Design review of the part shown in the three views and the two pictorial views. Dimensions are in mm from the part's minimum x, y and z. A direction names the side the tool comes from. Give positions to 0.01 mm unless a question says otherwise; leave off trailing zeros. Loops run counter-clockwise (first coordinate to the right, second up) from the corner with the lowest first, then second, coordinate; pieces in that order, holes last. Notation, with made-up numbers: (42.5, 64.5) -> (99.5, 64.5) arc R10 ccw to (99.5, 81.5) -> close; hole circle Ø9 at (4, -34). An arc over 180 degrees is marked (long way). Answer as CSV lines item,"result".
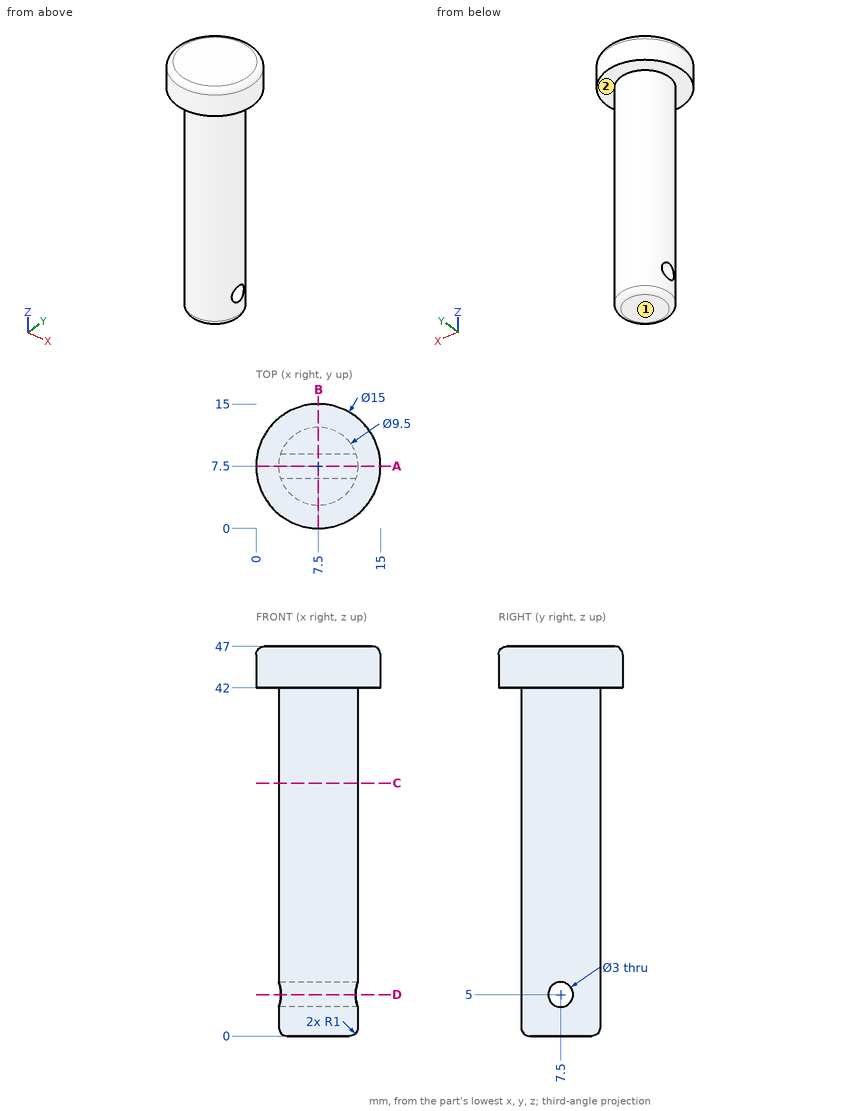
Q1. To check wall thickness, follow probe 1 along Z at (x, y) = (8, 7.5); probe 2 along Y at (x, z) = (7.75, 5); probe 3 along Y at (x, z) = (7.75, 23). State the ranges of each line that lie inside material, in increasing order. Write a range as from..to.
Filled sheet:
probe 1,"z = 0..3.5, 6.5..47"
probe 2,"y = 2.76..6, 9..12.24"
probe 3,"y = 2.76..12.24"
Q2. We need section C-C, the plane z = 30.5. State the section outline as (x, y) points, and give its area (3 significant figures).
Filled sheet:
outline,"circle Ø9.5 at (7.5, 7.5)"
area,"70.9 mm^2"
Q3. We need section A-A, the plane y = 7.5. State the section outline as (x, z) points, and give its area (3 significant figures).
Filled sheet:
outline,"(0, 42) -> (2.75, 42) -> (2.75, 6.5) -> (12.25, 6.5) -> (12.25, 42) -> (15, 42) -> (15, 46) arc R1 ccw to (14, 47) -> (1, 47) arc R1 ccw to (0, 46) -> close; (2.75, 1) arc R1 ccw to (3.75, 0) -> (11.25, 0) arc R1 ccw to (12.25, 1) -> (12.25, 3.5) -> (2.75, 3.5) -> close"
area,"445 mm^2"
Q4. We need section B-B, the plane x = 7.5. State the section outline as (y, z) points.
Filled sheet:
outline,"(0, 42) -> (2.75, 42) -> (2.75, 1) arc R1 ccw to (3.75, 0) -> (11.25, 0) arc R1 ccw to (12.25, 1) -> (12.25, 42) -> (15, 42) -> (15, 46) arc R1 ccw to (14, 47) -> (1, 47) arc R1 ccw to (0, 46) -> close; hole circle Ø3 at (7.5, 5)"
Q5. Clearance check with flat-ended pins moving along their axes: pin 1 Ø6 at (y, z) = (3.5, 8.5) entering from +X; pin 2 Ø5 at (x, z) = (12, 17) entering from -Y; pin 3 Ø6 at (y, z) = (8.5, 17) entering from +X; pin 4 Ø2.5 at (y, z) = (7.5, 5) entering from -X. State where each tip first meets the part, or that it passes through.
Filled sheet:
pin 1,"stops at x = 12.14"
pin 2,"stops at y = 3.19"
pin 3,"stops at x = 12.25"
pin 4,"passes through"
Q6. We need section D-D, the plane z = 5. State the section outline as (x, y) points.
Filled sheet:
outline,"(2.99, 6) arc R4.75 ccw to (12.01, 6) -> close; (2.99, 9) -> (12.01, 9) arc R4.75 ccw to start"
Q7. For the marked faces 1 and 2, list the 3-axis set-ups (+Z, -Z, +X, -X, +Y, -Y) from which the entire face can be reached by the end or side of a thin tool; tool diameter is ignored.
Filled sheet:
face 1,"-Z, +X, -X, +Y, -Y"
face 2,"-Z"
